```python
from build123d import *

# Parameters (mm, degrees)
P_IDAT_VYSUNUT_M1_DEPTH                           = 42.5
ODEBRAT_VYSUNUT_M1_DEPTH                          = 152.129911004
ODEBRAT_VYSUNUT_M1_DEPTH_BACK                     = 152.129911004
P_IDAT_VYSUNUT_M2_DEPTH                           = 9
ODEBRAT_VYSUNUT_M2_DEPTH                          = 135.652330095
ODEBRAT_VYSUNUT_M2_DEPTH_BACK                     = 135.652330095
V_LCOV_ZAHLOUBEN_PRO_M5_ROUBY_S_V_2_COUNT         = 2
V_LCOV_ZAHLOUBEN_PRO_M5_ROUBY_S_V_2_PITCH         = 27.950849719
V_LCOV_ZAHLOUBEN_PRO_M5_ROUBY_S_V_3_COUNT         = 2
V_LCOV_ZAHLOUBEN_PRO_M5_ROUBY_S_V_3_PITCH         = 27.950849719
V_LCOV_ZAHLOUBEN_PRO_M10_ROUBY_S_V_LC_D           = 10
V_LCOV_ZAHLOUBEN_PRO_M10_ROUBY_S_V_LC_CBORE_D     = 30
V_LCOV_ZAHLOUBEN_PRO_M10_ROUBY_S_V_LC_CBORE_DEPTH = 12
ZAOBLIT1_R                                        = 20


with BuildPart() as part:
    # Skica1 → Přidat vysunutím1 (new, symmetric)
    with BuildSketch(Plane.XY):
        Polygon((0, 0), (135, 0), (135, 12), (25, 12), (25, 65), (17.416697508, 65), align=None)
    extrude(amount=P_IDAT_VYSUNUT_M1_DEPTH, both=True)

    # Skica2 → Odebrat vysunutím1 (cut, two sides: drawn at the far end of the back side and taken through both)
    with BuildSketch(Plane(origin=(0, 12, 0), x_dir=(1, 0, 0), z_dir=(0, 1, 0)).offset(-ODEBRAT_VYSUNUT_M1_DEPTH_BACK)):
        with BuildLine():
            Line((-62.938175678, 293.50791206), (120.203054159, 42.5))
            ThreePointArc((120.203054159, 42.5), (134.922176639, 0.576231991), (124.027539054, -42.5))
            Line((124.027539054, -42.5), (-35.831632193, -308.940851505))
            Line((-35.831632193, -308.940851505), (584.976307558, -281.00825635))
            Line((584.976307558, -281.00825635), (557.869764074, 321.440507215))
            Line((557.869764074, 321.440507215), (-62.938175678, 293.50791206))
        make_face()
    extrude(amount=ODEBRAT_VYSUNUT_M1_DEPTH + ODEBRAT_VYSUNUT_M1_DEPTH_BACK, mode=Mode.SUBTRACT)

    # Skica3 → Přidat vysunutím2 (add)
    with BuildSketch(Plane(origin=(0, 12, 0), x_dir=(1, 0, 0), z_dir=(0, 1, 0))):
        with BuildLine():
            Line((25, 23.115200195), (58, 23.115200195))
            ThreePointArc((58, 23.115200195), (84, -2.884799805), (58, -28.884799805))
            Line((58, -28.884799805), (25, -28.884799805))
            Line((25, -28.884799805), (25, 23.115200195))
        make_face()
    extrude(amount=P_IDAT_VYSUNUT_M2_DEPTH)

    # Skica4 → Odebrat vysunutím2 (cut, two sides: drawn at the far end of the back side and taken through both)
    with BuildSketch(Plane(origin=(25, 0, 0), x_dir=(0, 0, -1), z_dir=(1, 0, 0)).offset(-ODEBRAT_VYSUNUT_M2_DEPTH_BACK)):
        with BuildLine():
            Line((15, 65), (15, 45))
            ThreePointArc((15, 45), (0, 30), (-15, 45))
            Line((-15, 45), (-15, 65))
            Line((-15, 65), (15, 65))
        make_face()
    extrude(amount=ODEBRAT_VYSUNUT_M2_DEPTH + ODEBRAT_VYSUNUT_M2_DEPTH_BACK, mode=Mode.SUBTRACT)

    # Skica9 → Válcové zahloubení pro M5 šrouby s válcovou hlavou zaoblenou1 (revolve, cut)
    with BuildSketch(Plane(origin=(25, 60, 0), x_dir=(0, 0, -1), z_dir=(0, 1, 0))):
        Polygon((0, 0), (0, 25), (2.5, 25), (2.5, 5), (5, 5), (5, 0.525), (5.525, 0), align=None)
    v_lcov_zahlouben_pro_m5_rouby_s_v_lco = revolve(axis=Axis((31.35, 60, 0), (-1, 0, 0)), mode=Mode.SUBTRACT)

    # V_lcov_ zahlouben_ pro M5 _rouby s v 2: Válcové zahloubení pro M5 šrouby s válcovou hlavou zaoblenou1 ×2
    with Locations(*[Vector(0, -0.1788854381999832, -0.9838699100999074) * (i * V_LCOV_ZAHLOUBEN_PRO_M5_ROUBY_S_V_2_PITCH) for i in range(1, V_LCOV_ZAHLOUBEN_PRO_M5_ROUBY_S_V_2_COUNT)]):
        add(v_lcov_zahlouben_pro_m5_rouby_s_v_lco, mode=Mode.SUBTRACT)

    # V_lcov_ zahlouben_ pro M5 _rouby s v 3: Válcové zahloubení pro M5 šrouby s válcovou hlavou zaoblenou1 ×2
    with Locations(*[Vector(0, -0.1788854381999834, 0.9838699100999074) * (i * V_LCOV_ZAHLOUBEN_PRO_M5_ROUBY_S_V_3_PITCH) for i in range(1, V_LCOV_ZAHLOUBEN_PRO_M5_ROUBY_S_V_3_COUNT)]):
        add(v_lcov_zahlouben_pro_m5_rouby_s_v_lco, mode=Mode.SUBTRACT)

    # Válcové zahloubení pro M10 šrouby s válcovou hlavou zaoblenou3 (through all)
    with Locations(Plane(origin=(0, 21, 0), x_dir=(1, 0, 0), z_dir=(0, 1, 0))):
        with Locations((58, -2.884799805)):
            CounterBoreHole(V_LCOV_ZAHLOUBEN_PRO_M10_ROUBY_S_V_LC_D / 2, V_LCOV_ZAHLOUBEN_PRO_M10_ROUBY_S_V_LC_CBORE_D / 2, V_LCOV_ZAHLOUBEN_PRO_M10_ROUBY_S_V_LC_CBORE_DEPTH)

    # Zaoblit1
    zaoblit1_edges = [part.edges().sort_by_distance(p)[0] for p in [
        (120.203054159, 6, -42.5),
        (124.027539054, 6, 42.5),
    ]]
    fillet(zaoblit1_edges, radius=ZAOBLIT1_R)


solid = part.part
```
Work out the finished part from the listing and answer in its coordinate system (mm). A direction names the side the tool comes from. Coordinates: 2 decimals unless noted, no trailing zeros. Loops run counter-clockwise (first coordinate to the right, second up) from the corner with the lowest first, then second, coordinate; pieces in that order, holes last.
1) Consider probe 1 along Z at (x, y) = (18.3, 55); probe 2 along Z at (x, y) = (22.9, 55); probe 3 along Y at (x, z) = (18.3, -27.5). Determine where each line is inside the solid, lowest interval first.
Results:
probe 1: z = -42.5 to -30, -25 to -15, 15 to 25, 30 to 42.5
probe 2: z = -42.5 to -32.5, -22.5 to -15, 15 to 22.5, 32.5 to 42.5
probe 3: y = 0 to 52.5, 57.5 to 65
2) For a pull along Y with two mould halves and no side action, classify faces 1 (the flat face through (67, 0, 1)), 2 (the cylindrical face through (119.44, 6.08, -39.58)), 3 (the cylindrical face through (16, 30, 0)), 4 (the cylindrical face through (22.269, 51.621, 31.185)) as +Y half, -Y half, draft (parallel to the pull), parting line (faces both ways), or undercut.
Results:
face 1: -Y half
face 2: draft
face 3: +Y half
face 4: undercut
3) For faces 5 (the flat face through (41, 16, -23.115)), 6 (the cylindrical face through (43.015, 15.084, 2.225)), 7 (the flat face through (20, 56, 25)), determine the directions among +Z, -Z, +X, -X, +Y, -Y from which every point of the face is accessible in a straight line to the end or side of a thin tool.
Results:
face 5: -Z, +X, +Y
face 6: +Y
face 7: +X
4) Section D-D (x = 107.5) is taken. Give the vertices of the cut face in (y, z), plus the area to 3 significant figures.
Results:
outline: (0, -42.5) - (12, -42.5) - (12, 42.5) - (0, 42.5) - close
area: 1,020 mm2
5) Section A-A (z = 0) is taken. Give the vertices of the cut face in (x, y).
Results:
outline: (0, 0) - (53.92, 0) - (53.92, 9) - (43.28, 9) - (43.28, 21) - (25, 21) - (25, 30) - (8.04, 30) - close; (62.08, 0) - (134.95, 0) - (134.95, 12) - (83.84, 12) - (83.84, 21) - (72.72, 21) - (72.72, 9) - (62.08, 9) - close
6) Section B-B (y = 37.5) is taken. Give the vertices of the cut face in (x, z).
Results:
outline: (10.05, -42.5) - (25, -42.5) - (25, -12.99) - (10.05, -12.99) - close; (10.05, 12.99) - (25, 12.99) - (25, 42.5) - (10.05, 42.5) - close
7) Section C-C (y = 7) is taken. Give the vertices of the cut face in (x, z).
Results:
outline: (1.88, -42.5) - (109.04, -42.5) arc R20 ccw to (126.94, -31.41) arc R77 ccw to (130.3, 29.38) arc R20 ccw to (111.52, 42.5) - (1.88, 42.5) - close; hole circle Ø10 at (58, 2.88)
8) Flat-ended cylindrical pins translate along their axes: pin 1 (6 mm diameter, centred on y = 55, z = 27.5, fed in from -X); pin 2 (10 mm diameter, centred on y = 18, z = -9.5, fed in from +X); pin 3 (12 mm diameter, centred on y = 10, z = 29, fed in from +X). Find the tip coordinate at first contact, or state that the pin passes through.
Results:
pin 1: stops at x = 13.93
pin 2: stops at x = 82.93
pin 3: stops at x = 132.33
